Build history of the part. All positions in model axes, mm. A direction names the side the tool comes from. Round coordinates to 2 decimals unless told otherwise and drop trailing zeros. Loops run counter-clockwise (first coordinate to the right, second up) from the corner with the lowest first, then second, coordinate; pieces in that order, holes last.
from build123d import *

# Parameters (mm, degrees)
BOSS_EXTRUDE1_DEPTH = 10
SKETCH3_R           = 2.25
CUT_EXTRUDE1_DEPTH  = 19.874586088
SKETCH4_W           = 9
SKETCH4_H           = 17.100076188
CUT_EXTRUDE2_DEPTH  = 5.25
FILLET1_R           = 5


with BuildPart() as part:
    # Sketch1 → Boss-Extrude1 (new, symmetric)
    with BuildSketch(Plane(origin=(0, 0, 0), x_dir=(0, 0, -1), z_dir=(1, 0, 0))):
        Polygon((-9.5, 3), (-9.5, 4.7), (-10.5, 4.7), (-12.5, 2.7), (-12.5, -2.7), (-10.5, -4.7), (-9.5, -4.7), (-9.5, -3), (-7, -3), (-7, -10), (0, -10), (0, 10), (-7, 10), (-7, 3), align=None)
    extrude(amount=BOSS_EXTRUDE1_DEPTH, both=True)

    # Sketch3 → Cut-Extrude1 (cut, through all)
    with BuildSketch(Plane(origin=(0, 0, 0), x_dir=(-1, 0, 0), z_dir=(0, 0, -1))):
        Circle(SKETCH3_R)
    extrude(amount=-CUT_EXTRUDE1_DEPTH, mode=Mode.SUBTRACT)

    # Sketch4 → Cut-Extrude2 (cut, symmetric)
    with BuildSketch(Plane(origin=(0, 0, 0), x_dir=(0, 0, -1), z_dir=(1, 0, 0))):
        with Locations((-12.5, 0)):
            Rectangle(SKETCH4_W, SKETCH4_H)
    extrude(amount=CUT_EXTRUDE2_DEPTH, both=True, mode=Mode.SUBTRACT)

    # Fillet1
    fillet1_edges = [part.edges().sort_by_distance(p)[0] for p in [
        (10, -10, 3.5),
        (-10, 10, 3.5),
        (-10, -10, 3.5),
        (10, 10, 3.5),
    ]]
    fillet(fillet1_edges, radius=FILLET1_R)


solid = part.part
(1) Slice it at C-C on z = 1.5. List the corners of the cut face in (x, y).
Responses:
outline: (-10, -5) arc R5 ccw to (-5, -10) - (5, -10) arc R5 ccw to (10, -5) - (10, 5) arc R5 ccw to (5, 10) - (-5, 10) arc R5 ccw to (-10, 5) - close; hole circle Ø4.5 at (0, 0)
(2) Probe line 1 (Y direction, x = 0, z = 2.5); line 2 (X direction, y = 0.5, z = 9.75); line 3 (Z direction, x = -3.25, y = 2). List the from-to ranges inside material, lowest first.
Responses:
line 1: y = -10 to -2.25, 2.25 to 10
line 2: x = -10 to -5.25, 5.25 to 10
line 3: z = 0 to 8
(3) Pin check, flat tips, straight feed: P1, Ø1.5, axis at y = 6, z = 4, coming from the -X side; P2, Ø0.8, axis at x = -6.5, z = 10, coming from the -Y side; P3, Ø0.8, axis at x = -7.5, z = 10, coming from the +Y side. Stop position of each tip, or through.
Responses:
P1: stops at x = -9.99
P2: stops at y = -4.7
P3: stops at y = 4.7
(4) Which spindle directions (+Z, -Z, +X, -X, +Y, -Y) get a long thin tool onto all of the face, cutting with end or side? Do faces 5 (the face through (0.1, 3, 7.7)), 6 (the face through (-8, -4.7, 10)), 7 (the face through (8, 4.7, 10)). Say none if no direction does.
Responses:
face 5: +X, -X, +Y
face 6: +Z, +X, -X, -Y
face 7: +Z, +X, -X, +Y
(5) Slice it at A-A on y = 0. List the corners of the cut face in (x, z).
Responses:
outline: (-10, 0) - (-2.25, 0) - (-2.25, 8) - (-5.25, 8) - (-5.25, 12.5) - (-10, 12.5) - close; (2.25, 0) - (10, 0) - (10, 12.5) - (5.25, 12.5) - (5.25, 8) - (2.25, 8) - close
(6) Slice it at D-D on x = -3. List the corners of the cut face in (y, z).
Responses:
outline: (-10, 0) - (10, 0) - (10, 7) - (3, 7) - (3, 8) - (-3, 8) - (-3, 7) - (-10, 7) - close
(7) Slice it at B-B on x = 0. List the corners of the cut face in (y, z).
Responses:
outline: (-10, 0) - (-2.25, 0) - (-2.25, 8) - (-3, 8) - (-3, 7) - (-10, 7) - close; (2.25, 0) - (10, 0) - (10, 7) - (3, 7) - (3, 8) - (2.25, 8) - close
(8) Pull direction Z, two halves, no side cores. Call faces 1 (the face through (-7.6, 3.7, 11.5)), 2 (the face through (-9, 8, 4)), 3 (the face through (-8, -4, 9.5)), 4 (the face through (8, 4, 9.5)): +Z half, -Z half, draft (parallel to the pull), parting line (faces both ways), or undercut.
Responses:
face 1: +Z half
face 2: draft
face 3: undercut
face 4: undercut
